```python
from build123d import *

# Parameters (mm, degrees)
F1_DEPTH = 6.35
F2_R     = 1.8288
F3_R     = 1.8288
F4_DEPTH = 6.005883
F5_R     = 2.54


with BuildPart() as f1:
    # F0 (on Top) → F1 (new body)
    with BuildSketch(Plane.XY):
        with BuildLine():
            ThreePointArc((0, 13.335), (13.335, 0), (0, -13.335))
            Line((0, -13.335), (0, -31.446429))
            Line((0, -31.446429), (6.005883, -31.446429))
            Line((6.005883, -31.446429), (6.005883, -18.746429))
            ThreePointArc((6.005883, -18.746429), (19.685, 0), (6.005883, 18.746429))
            Line((6.005883, 18.746429), (6.005883, 31.446429))
            Line((6.005883, 31.446429), (0, 31.446429))
            Line((0, 31.446429), (0, 13.335))
        make_face()
    extrude(amount=F1_DEPTH)

    # F2 (on face) + F3 (on face) → F4 (cut, through all)
    with BuildSketch(Plane.YZ.offset(6.005883)):
        with Locations((-25.096429, 3.175)):
            Circle(F2_R)
    with BuildSketch(Plane.YZ.offset(6.005883)):
        with Locations((25.096429, 3.175)):
            Circle(F3_R)
    extrude(amount=-F4_DEPTH, mode=Mode.SUBTRACT)

    # F5
    f5_edges = [f1.edges().sort_by_distance(p)[0] for p in [
        (6.005883, -18.746429, 3.175),
        (6.005883, 18.746429, 3.175),
    ]]
    fillet(f5_edges, radius=F5_R)


solid = f1.part
```
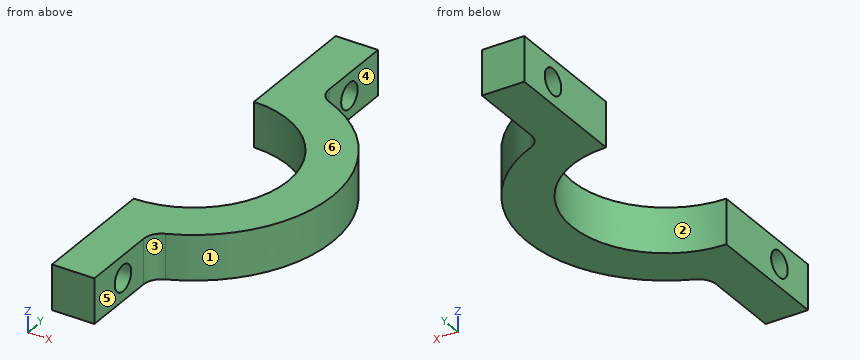
Source: CAD feature listing. Evaluate the final solid. Frame: model axes, mm. Face numbers are marked on the shaded views. A direction names the side the tool comes from. Give positions to 0.01 mm unless a question says otherwise; leave off trailing zeros. Loops run counter-clockwise (first coordinate to the right, second up) from the corner with the lowest first, then second, coordinate; pieces in that order, holes last. Notation, with made-up numbers: (-32, 29) -> (5, 29) arc R15 ccw to (5, 57) -> close; hole circle Ø9 at (24.5, -7.5). An arc over 180 degrees is marked (long way). Use a Markdown table: item, result. Add a question column.
(1) Section query C-C (x = 10). Output: boundary loops of the cut face in (y, z).
(2) Ray query, line 1 (Y direction, x = 2, z = 4.5); line 2 (Y direction, x = 5.25, z = 2); line 3 (Y direction, x = 7, z = 0.5). Return the intervals inside material, ascending.
(3) Section query B-B (x = 4.25). Output: boundary loops of the cut face in (y, z) (3 decimals).
(4) Pull-direction query (Y, two-part tool) for the marked faces 1, 2 and 3; classes: +Y half, -Y half, draft (parallel to the pull), parting line (faces both ways), or undercut.
(5) Access query for the marked faces 4, 5 and 6. Directions: +Z, -Z, +X, -X, +Y, -Y. A direction counts if a zero-diameter tool reaches every point of the face in a straight line with its end or side. Return the directions, or none.
(6) Section query D-D (y = 0). Output: boundary loops of the cut face in (x, z) (3 decimals).
(7) First-contact query: pin 1 Ø1 at (x, z) = (7, 4.5) entering from -Y; pin 2 Ø1 at (y, z) = (-6, 2.5) entering from +X. Flat tips, straight axial feed; report the tip coordinate or a pass-through.
(8) Section query A-A (x = 1.5). Output: boundary loops of the cut face in (y, z) (3 decimals).
Checked values:
| question | item | result |
|---|---|---|
| 1 | outline | (-16.96, 0) -> (-8.82, 0) -> (-8.82, 6.35) -> (-16.96, 6.35) -> close; (8.82, 0) -> (16.96, 0) -> (16.96, 6.35) -> (8.82, 6.35) -> close |
| 2 | line 1 | -31.45 to -26.36, -23.84 to -13.18, 13.18 to 23.84, 26.36 to 31.45 |
| 2 | line 2 | -31.45 to -26.5, -23.7 to -12.26, 12.26 to 23.7, 26.5 to 31.45 |
| 2 | line 3 | -18.5 to -11.35, 11.35 to 18.5 |
| 3 | outline | (-31.446, 0) -> (-12.64, 0) -> (-12.64, 6.35) -> (-31.446, 6.35) -> close; (12.64, 0) -> (31.446, 0) -> (31.446, 6.35) -> (12.64, 6.35) -> close; hole circle Ø3.658 at (-25.096, 3.175); hole circle Ø3.658 at (25.096, 3.175) |
| 4 | face 1 | parting line |
| 4 | face 2 | undercut |
| 4 | face 3 | -Y half |
| 5 | face 4 | +Z, -Z, +X, +Y |
| 5 | face 5 | +Z, -Z, +X, -Y |
| 5 | face 6 | +Z, +X, -X, +Y, -Y |
| 6 | outline | (13.335, 0) -> (19.685, 0) -> (19.685, 6.35) -> (13.335, 6.35) -> close |
| 7 | pin 1 | y = -19.01 |
| 7 | pin 2 | x = 18.9 |
| 8 | outline | (-31.446, 0) -> (-13.25, 0) -> (-13.25, 6.35) -> (-31.446, 6.35) -> close; (13.25, 0) -> (31.446, 0) -> (31.446, 6.35) -> (13.25, 6.35) -> close; hole circle Ø3.658 at (-25.096, 3.175); hole circle Ø3.658 at (25.096, 3.175) |
